```python
from build123d import *

# Parameters (mm, degrees)
SKETCH1_W           = 35
SKETCH1_H           = 35
SKETCH1_R           = 1.45
SKETCH1_R_2         = 1.6
BOSS_EXTRUDE1_DEPTH = 13
SHELL1_T            = -3
SKETCH2_W           = 29
SKETCH2_H           = 40.523208079
CUT_EXTRUDE1_DEPTH  = 10
FILLET1_R           = 1.5
SKETCH4_R           = 1.45
BOSS_EXTRUDE3_DEPTH = 2
FILLET2_R           = 1


with BuildPart() as part:
    # Sketch1 → Boss-Extrude1 (new body)
    with BuildSketch(Plane(origin=(0, 0, 0), x_dir=(1, 0, 0), z_dir=(0, 1, 0))):
        Rectangle(SKETCH1_W, SKETCH1_H)
        with Locations(Location((6.21, 7.5, 0), (0, 0, 90))):
            Circle(SKETCH1_R, mode=Mode.SUBTRACT)
        with Locations(Location((0, 7.5, 0), (0, 0, 90))):
            Circle(SKETCH1_R_2, mode=Mode.SUBTRACT)
        with Locations(Location((-6.21, 7.5, 0), (0, 0, 90))):
            Circle(SKETCH1_R, mode=Mode.SUBTRACT)
        with Locations(Location((-6.21, -4.92, 0), (0, 0, 90))):
            Circle(SKETCH1_R, mode=Mode.SUBTRACT)
        with Locations(Location((6.21, -4.92, 0), (0, 0, 90))):
            Circle(SKETCH1_R, mode=Mode.SUBTRACT)
        with Locations(Location((-6.21, -12.5, 0), (0, 0, 90))):
            Circle(SKETCH1_R_2, mode=Mode.SUBTRACT)
        with Locations(Location((6.21, -12.5, 0), (0, 0, 90))):
            Circle(SKETCH1_R_2, mode=Mode.SUBTRACT)
    extrude(amount=BOSS_EXTRUDE1_DEPTH)

    # Shell1
    shell1_openings = [part.faces().sort_by_distance(p)[0] for p in [
        (0, 13, -0.090817289),
    ]]
    offset(amount=SHELL1_T, openings=shell1_openings, kind=Kind.INTERSECTION)

    # Sketch2 → Cut-Extrude1 (cut)
    with BuildSketch(Plane(origin=(0, 13, 0), x_dir=(1, 0, 0), z_dir=(0, 1, 0))):
        with Locations((0, 4.76160404)):
            Rectangle(SKETCH2_W, SKETCH2_H)
    extrude(amount=-CUT_EXTRUDE1_DEPTH, mode=Mode.SUBTRACT)

    # Fillet1
    fillet1_edges = [part.edges().sort_by_distance(p)[0] for p in [
        (-17.5, 6.5, -17.5),
        (17.5, 6.5, -17.5),
        (17.5, 6.5, 17.5),
        (-17.5, 6.5, 17.5),
    ]]
    fillet(fillet1_edges, radius=FILLET1_R)

    # Sketch4 → Boss-Extrude3 (add)
    # profile 1 of 2: a face of its own
    with BuildSketch(Plane(origin=(0, 11, 0), x_dir=(1, 0, 0), z_dir=(0, 1, 0))):
        with BuildLine():
            Line((-17.5, -3.5), (-21.5, -3.5))
            ThreePointArc((-21.5, -3.5), (-25, 0), (-21.5, 3.5))
            Line((-21.5, 3.5), (-17.5, 3.5))
            Line((-17.5, 3.5), (-17.5, -3.5))
        make_face()
        with Locations(Location((-21.5, 0, 0), (0, 0, 270))):
            Circle(SKETCH4_R, mode=Mode.SUBTRACT)
    # profile 2 of 2: a face of its own
    with BuildSketch(Plane(origin=(0, 11, 0), x_dir=(1, 0, 0), z_dir=(0, 1, 0))):
        with BuildLine():
            Line((17.5, 3.5), (21.5, 3.5))
            ThreePointArc((21.5, 3.5), (25, 0), (21.5, -3.5))
            Line((21.5, -3.5), (17.5, -3.5))
            Line((17.5, -3.5), (17.5, 3.5))
        make_face()
        with Locations(Location((21.5, 0, 0), (0, 0, 270))):
            Circle(SKETCH4_R, mode=Mode.SUBTRACT)
    extrude(amount=-BOSS_EXTRUDE3_DEPTH)

    # Fillet2
    fillet2_edges = [part.edges().sort_by_distance(p)[0] for p in [
        (-17.5, 9, 0),
        (-17.5, 10, -3.5),
        (-17.5, 10, 3.5),
        (17.5, 9, 0),
        (17.5, 10, 3.5),
        (17.5, 10, -3.5),
    ]]
    fillet(fillet2_edges, radius=FILLET2_R)


solid = part.part
```
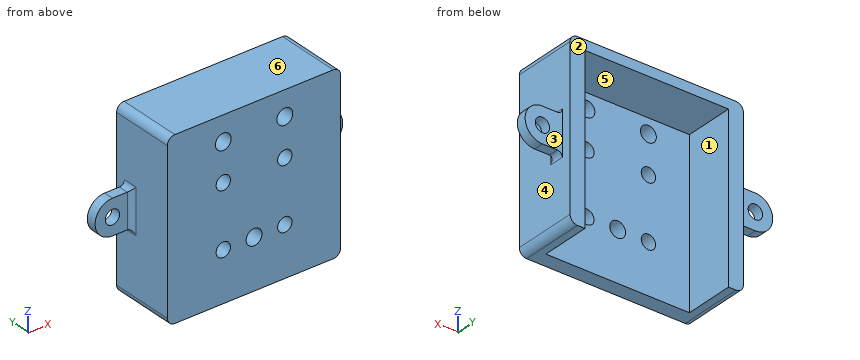
Work out the finished part from the listing and answer in its coordinate system (mm). Face numbers are marked on the shaded views. A direction names the side the tool comes from. Round coordinates to 2 decimals unless told otherwise and drop trailing zeros. Loops run counter-clockwise (first coordinate to the right, second up) from the corner with the lowest first, then second, coordinate; pieces in that order, holes last. Notation, with made-up numbers: M 78.5,-24 L 130.5,-24 A25 ccw 130.5,11 Z; hole C 81,61.25 d11. An arc over 180 degrees is marked long. One line per question, with ' | ' between items.
Q1. Consider line 1 along X through (y, z) = (10, 0); line 2 along X through (y, z) = (0.7, 4.92); line 3 along X through (y, z) = (1.7, 12.5). Determine where each line is inside the solid, lowest interval first. Write a range as from..to.
Conclusion:
line 1: x = -25..-22.95, -20.05..-14.5, 14.5..20.05, 22.95..25 | line 2: x = -17.5..-7.66, -4.76..4.76, 7.66..17.5 | line 3: x = -17.5..-7.81, -4.61..4.61, 7.81..17.5
Q2. A tool of negligible diameter and unlimited length cuts with its end or side. For the marked faces 1, 2 and 3, from which of +Z, -Z, +X, -X, +Y, -Y can it reach the whole face along a straight path? Write none if from no direction.
Conclusion:
face 1: -Z, +Y | face 2: +Z, -Z, +X, -X, +Y | face 3: +Z, -Z, +X, +Y
Q3. The mould has two halves that part along X. Classify the marked faces 4, 5 and 6: +X half, -X half, draft (parallel to the pull), parting line (faces both ways), or undercut.
Conclusion:
face 4: +X half | face 5: undercut | face 6: draft
Q4. Find section D-D, the plane x = -6.21. Give the vertices of the cut face in (y, z).
Conclusion:
outline: M 0,-17.5 L 3,-17.5 L 3,-8.95 L 0,-8.95 Z; M 0,-6.05 L 3,-6.05 L 3,3.47 L 0,3.47 Z; M 0,6.37 L 3,6.37 L 3,10.9 L 0,10.9 Z; M 0,14.1 L 3,14.1 L 3,15.5 L 13,15.5 L 13,17.5 L 0,17.5 Z
Q5. Find section B-B, the plane y = 10.5. Give the vertices of the cut face in (x, z), then the cut area to 3 significant figures.
Conclusion:
outline: M -21.5,-3.5 L -18.5,-3.5 A1 cw -17.5,-4.5 L -17.5,-16 A1.5 ccw -16,-17.5 L -14.5,-17.5 L -14.5,15.5 L 14.5,15.5 L 14.5,-17.5 L 16,-17.5 A1.5 ccw 17.5,-16 L 17.5,-4.5 A1 cw 18.5,-3.5 L 21.5,-3.5 A3.5 ccw 21.5,3.5 L 18.5,3.5 A1 cw 17.5,4.5 L 17.5,16 A1.5 ccw 16,17.5 L -16,17.5 A1.5 ccw -17.5,16 L -17.5,4.5 A1 cw -18.5,3.5 L -21.5,3.5 A3.5 ccw Z; hole C -21.5,0 d2.9; hole C 21.5,0 d2.9 | area: 348 mm2
Q6. Find section A-A, the plane x = 0. Give the vertices of the cut face in (y, z).
Conclusion:
outline: M 0,-17.5 L 3,-17.5 L 3,-9.1 L 0,-9.1 Z; M 0,-5.9 L 3,-5.9 L 3,15.5 L 13,15.5 L 13,17.5 L 0,17.5 Z
Q7. Each of these flat-tipped pins is pushed along its axis until it touches: pin 1 Ø4 at (x, z) = (23, 0) entering from +Y; pin 2 Ø3 at (x, z) = (21.5, 0.5) entering from -Y; pin 3 Ø1 at (y, z) = (9.5, 12.5) entering from -X; pin 4 Ø1.7 at (x, z) = (-6.21, -7.5) entering from -Y. Where does it stop, or does it pass through?
Conclusion:
pin 1: stops at y = 11 | pin 2: stops at y = 9 | pin 3: stops at x = -17.5 | pin 4: passes through
Q8. Find section C-C, the plane z = -7.5. Give the vertices of the cut face in (x, y).
Conclusion:
outline: M -17.5,0 L -7.66,0 L -7.66,3 L -14.5,3 L -14.5,13 L -17.5,13 Z; M -4.76,0 L -1.6,0 L -1.6,3 L -4.76,3 Z; M 1.6,0 L 4.76,0 L 4.76,3 L 1.6,3 Z; M 7.66,0 L 17.5,0 L 17.5,13 L 14.5,13 L 14.5,3 L 7.66,3 Z
